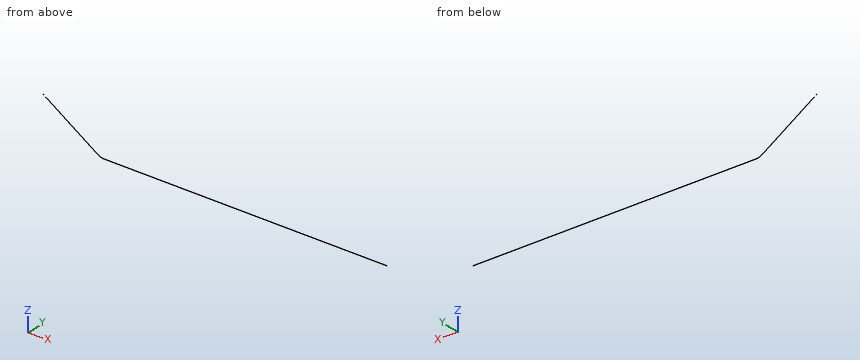
```python
from build123d import *

# Parameters (mm, degrees)
SWEEP1_PROFILE_R    = 0.25
SKETCH6_R           = 0.1
BOSS_EXTRUDE1_DEPTH = 5


with BuildPart() as part:
    # Sweep1: sweep along a path in Sketch2
    with BuildLine(Plane(origin=(0, 0, 0), x_dir=(1, 0, 0), z_dir=(0, 1, 0))) as sweep1_path:
        Line((500, 20), (0, 20))
        ThreePointArc((0, 20), (-5.730491055, 19.161457989), (-10.98045636, 16.716147227))
        Line((-10.98045636, 16.716147227), (-103.755073472, -44.22538557))
    # Sweep1 profile (on start of the path) → Sweep1 (sweep)
    with BuildSketch(Plane(origin=(500, 0, -20), x_dir=(0, 0, -1), z_dir=(-1, 0, 0))):
        Circle(SWEEP1_PROFILE_R)
    sweep(path=sweep1_path.line)

    # Sketch6 → Boss-Extrude1 (add)
    with BuildSketch(Plane(origin=(-92.774617112, 0, 60.941532798), x_dir=(0.5490228179981329, 0, 0.8358073613682695), z_dir=(-0.8358073613682695, 0, 0.5490228179981329))):
        with Locations((-20, 0)):
            Circle(SKETCH6_R)
    extrude(amount=BOSS_EXTRUDE1_DEPTH)


solid = part.part
```
Read the model definition and answer for the solid it produces. Units are mm, in the model's axes. Give positions to 0.01 mm unless a question says otherwise; leave off trailing zeros. Order: outer loops, then holes, each group sorted by start corner. A loop starts at its lowest first (then second) coordinate and runs counter-clockwise, first axis right, second up. Notation, with made-up numbers: (74, 37.25) -> (122, 37.25) arc R10 cw to (122, 50.25) -> close; hole circle Ø3 at (-38, 22.25). An arc over 180 degrees is marked (long way). One line per item, written item: value. Start each with the question number.
(1) Straight lines are drawn through the part: L1, parallel to Z at x = 457.5, y = -0.05; L2, parallel to Z at x = 253, y = 0.2; L3, parallel to X at y = 0.15, z = 31. For each, find the intervals that lie inside material, in ascending order.
(2) The part is cut by section B-B (x = 298). Determine the outline of the cut face in (y, z), and give its area (3 significant figures).
(3) The part is cut by section A-A (y = 0). Determine the outline of the cut face in (x, z), and give its area (3 significant figures).
Taken from the geometry:
1. L1: -20.24 to -19.76
1. L2: -20.15 to -19.85
1. L3: -83.99 to -83.26
2. outline: circle Ø0.5 at (0, -20)
2. area: 0.196 mm^2
3. outline: (-107.99, 46.89) -> (-103.81, 44.14) -> (-103.89, 44.02) -> (-11.12, -16.93) arc R20.25 ccw to (0, -20.25) -> (500, -20.25) -> (500, -19.75) -> (0, -19.75) arc R19.75 cw to (-10.84, -16.51) -> (-103.62, 44.43) -> (-103.7, 44.31) -> (-107.88, 47.05) -> close
3. area: 312 mm^2
